Can you work these out from the model? Positions are in its coordinate system, mm. Face numbers are marked on the shaded views. Round coordinates to 2 decimals unless told otherwise and drop trailing zeros. Write each loop counter-clockwise with the first axis right and the second up, starting at its lowest first coordinate (ties: lowest second). Pieces come first, ordered by that corner, then holes. Notation, with made-up numbers: M 48.25,-17 L 88.25,-17 A9 ccw 88.25,-4 Z; hole C 19,28 d6. An arc over 180 degrees is marked long. Answer as a JSON object with one key per item and string values. Group by question number.
1) Suppose I cut it at A-A, the plane z = 0. Write out the boundary of the cut face in (x, y), and give its area (3 significant figures).
2) Please list where these lines run through material, in increasing order: L1, parallel to X at y = -0.25, z = -0.8; L2, parallel to Y at x = -1.5, z = -0.4; L3, parallel to X at y = -1, z = -1.3. Write a range as [from, to].
3) I'm going to push a flat-ended pin straight in: pin 1 Ø5 at (x, y) = (0, 0) entering from +Z. Where does the tip first touch, or does it pass through?
4) If we mould it in two halves opening along X, with no side actions, what happens to the marked faces 1, 2 and 3? For each: +X half, -X half, draft (parallel to the pull), parting line (faces both ways), or undercut.
from build123d import *

# Parameters (mm, degrees)
BOSS_EXTRUDE1_DEPTH = 1.651


with BuildPart() as part:
    # Sketch1 → Boss-Extrude1 (new body, symmetric)
    with BuildSketch(Plane(origin=(0, 1.651, 0), x_dir=(-1, 0, 0), z_dir=(0, 0, -1))):
        Polygon((2.749630657, 3.1115), (-2.749630657, 3.1115), (-5.499261314, -1.651), (-2.749630657, -6.4135), (2.749630657, -6.4135), (5.499261314, -1.651), align=None)
    extrude(amount=BOSS_EXTRUDE1_DEPTH, both=True)

    # Sketch2 → Cut-Revolve1 (revolve, cut)
    with BuildSketch(Plane(origin=(0, 0, 0), x_dir=(-1, 0, 0), z_dir=(0, 1, 0))):
        Polygon((-5.499261314, -1.225630657), (-5.499261314, -1.651), (-4.7625, -1.651), align=None)
    cut_revolve1 = revolve(axis=Axis((0, 0, 0), (0, 0, -1)), mode=Mode.SUBTRACT)

    # Sketch4 → Cut-Revolve3 (revolve, cut)
    with BuildSketch(Plane(origin=(0, 0, 0), x_dir=(1, 0, 0), z_dir=(0, 1, 0))):
        Polygon((2.413, 1.651), (0, 1.651), (0, -1.2192), (1.9812, -1.2192), (1.9812, 1.2192), align=None)
    cut_revolve3 = revolve(axis=Axis((0, 0, -1.651), (0, 0, 1)), mode=Mode.SUBTRACT)

    # Mirror1: Cut-Revolve1, Cut-Revolve3 across plane
    add(cut_revolve1.mirror(Plane.XY), mode=Mode.SUBTRACT)
    add(cut_revolve3.mirror(Plane.XY), mode=Mode.SUBTRACT)


solid = part.part
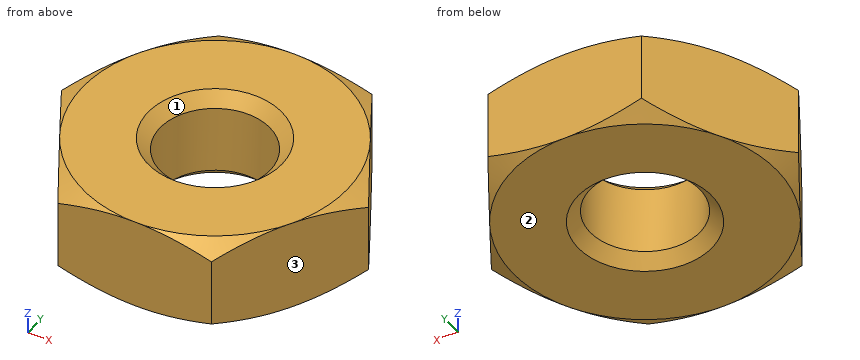
Results:
{
 "1": {"outline": "M -5.5,0 L -2.75,-4.76 L 2.75,-4.76 L 5.5,0 L 2.75,4.76 L -2.75,4.76 Z; hole C 0,0 d3.96", "area": "66.2 mm^2"},
 "2": {"L1": "[-5.35, -1.97], [1.97, 5.35]", "L2": "[-4.76, -1.29], [1.29, 4.76]", "L3": "[-4.92, -1.8], [1.8, 4.92]"},
 "3": {"pin 1": "z = 1.65"},
 "4": {"face 1": "undercut", "face 2": "draft", "face 3": "+X half"}
}
